```python
from build123d import *

# Parameters (mm, degrees)
F1_R     = 19
F2_DEPTH = 35.5
F0_R     = 1.625
F3_DEPTH = 8
F4_R     = 10
F5_DEPTH = 5
F6_R     = 3
F7_DEPTH = 12


with BuildPart() as f2:
    # F1 (on Front) → F2 (new body)
    with BuildSketch(Plane.XZ):
        Circle(F1_R)
    extrude(amount=-F2_DEPTH)

    # F0 (on Front) → F3 (cut)
    with BuildSketch(Plane.XZ):
        with Locations((15, 0)):
            Circle(F0_R)
        with Locations((-7.5, 12.990381)):
            Circle(F0_R)
        with Locations((-7.5, -12.990381)):
            Circle(F0_R)
    extrude(amount=-F3_DEPTH, mode=Mode.SUBTRACT)

    # F4 (on face) → F5 (join)
    with BuildSketch(Plane.XZ):
        Circle(F4_R)
    extrude(amount=F5_DEPTH)

    # F6 (on face) → F7 (join)
    with BuildSketch(Plane.XZ.offset(5)):
        Circle(F6_R)
    extrude(amount=F7_DEPTH)


solid = f2.part
```
Verification items for the finished model (mm, model axes). A direction names the side the tool comes from. Round coordinates to 2 decimals unless told otherwise and drop trailing zeros. Write each loop counter-clockwise with the first axis right and the second up, starting at its lowest first coordinate (ties: lowest second). Pieces come first, ordered by that corner, then holes. Notation, with made-up numbers: (38, -30) -> (95, -30) arc R15 cw to (95, -19) -> close; hole circle Ø5 at (29.5, -14). An arc over 180 degrees is marked (long way). Write each question's results on one line, items separated by ' | '. Start each with the question number.
1. Cross-section at C-C (y = 17.5). Enter the section's corners in (x, z).
2. Depth check by flat-ended pin: P1, Ø1.5, axis at y = 26.5, z = 14, coming from the +X side; P2, Ø1.6, axis at x = 15, z = 0, coming from the -Y side; P3, Ø2, axis at y = 4, z = -11, coming from the -X side. Enter the tip coordinate at first touch or a pass-through.
3. Material ranges on probe 1 along Z at (x, y) = (-7.5, 1.75); probe 2 along Z at (x, y) = (-7, 6); probe 3 along Y at (x, z) = (11.5, 10.5), recorded low to high. Write a range as from..to.
4. Set-up check for faces 1 (the flat face through (0, -17, 0)), 2 (the cylindrical face through (-9.123, 3.944, 13.062)): record each of +Z, -Z, +X, -X, +Y, -Y from which the full face is reachable in a straight line by a thin tool's end or side.
5. Cross-section at A-A (z = 0). Enter the section's corners in (x, y) (3 decimals).
6. Cross-section at D-D (z = 9). Enter the section's corners in (x, y).
7. Draft check along X on faces 3 (the flat face through (15, 8, 0)), 4 (the cylindrical face through (8.767, 17.502, -16.856)), 5 (the flat face through (0, 35.5, 0)). Enter one of: +X half, -X half, draft (parallel to the pull), parting line (faces both ways), or undercut.
8. Cross-section at B-B (x = 0). Enter the section's corners in (y, z).
Solutions:
1) outline: circle Ø38 at (0, 0)
2) P1: stops at x = 13.62 | P2: stops at y = 8 | P3: stops at x = -16.16
3) probe 1: z = -17.46..-14.62, -11.37..11.37, 14.62..17.46 | probe 2: z = -17.66..-14.54, -11.44..11.44, 14.54..17.66 | probe 3: y = 0..35.5
4) face 1: +Z, -Z, +X, -X, -Y | face 2: -Y
5) outline: (-19, 0) -> (-10, 0) -> (-10, -5) -> (-3, -5) -> (-3, -17) -> (3, -17) -> (3, -5) -> (10, -5) -> (10, 0) -> (13.375, 0) -> (13.375, 8) -> (16.625, 8) -> (16.625, 0) -> (19, 0) -> (19, 35.5) -> (-19, 35.5) -> close
6) outline: (-16.73, 0) -> (-4.36, 0) -> (-4.36, -5) -> (4.36, -5) -> (4.36, 0) -> (16.73, 0) -> (16.73, 35.5) -> (-16.73, 35.5) -> close
7) face 3: undercut | face 4: parting line | face 5: draft
8) outline: (-17, -3) -> (-5, -3) -> (-5, -10) -> (0, -10) -> (0, -19) -> (35.5, -19) -> (35.5, 19) -> (0, 19) -> (0, 10) -> (-5, 10) -> (-5, 3) -> (-17, 3) -> close
